Autodesk Inventor part; units mm, degrees
ref_plane "Lock Pin Hole Plane" through (0, 0, 12.7) normal (0, 0, 1) x (1, 0, 0)
ref_plane "YZ Plane" through (0, 0, 0) normal (1, 0, 0) x (0, 1, 0)
ref_plane "XZ Plane" through (0, 0, 0) normal (0, 1, 0) x (-1, 0, 0)
sketch "Sketch1" plane through (0, 0, 0) normal (1, 0, 0) x (0, 1, 0)
  circle A0 centre (0, 0) radius 6.19 construction
  circle A1 centre (0, 0) radius 10
  dimension "d0" = 20
  dimension "d1" = 3.81
extrude "Main Shaft" add sketch "Sketch1" against normal blind 50.8
sketch "Sketch2" plane through (0, 0, 0) normal (1, 0, 0) x (0, 0, -1)
  circle A0 centre (0, 0) radius 30
  dimension "d4" = 60
extrude "CV Flange" add sketch "Sketch2" along normal blind 5
sketch "Sketch3" plane through (5, 0, 0) normal (1, 0, 0) x (0, 0, -1)
  circle A0 centre (0, 20) radius 5
  circle A1 centre (0, 0) radius 20 construction
  line L0 (0, 0) -> (0, 20) construction
  dimension "d7" = 40
  dimension "d8" = 10
extrude "CV Bolt Hole" cut sketch "Sketch3" against normal up to surface (5 mm away)
pattern_circular "CV Bolt Pattern" count 6 over 360 about axis through (-10, 0, 0) along (1, 0, 0) of "CV Bolt Hole"
chamfer "Weld_Chamfer" distance 2 angle 45 1 edges at (0, -10, 0)
ref_plane "Lock Pin Hole Plane" through (0, 0, 12.7) normal (0, 0, 1) x (1, 0, 0)
sketch "Sketch5" plane through (-50.8, 0, 0) normal (-1, 0, 0) x (0, 0, 1)
  line L0 (-20, 0) -> (15, 0) construction
  line L1 (0, 14) -> (0, -14) construction
  arc A0 (-13, 2) -> (-13, -2) centre (-13, 0) ccw
  arc A1 (-7, -2) -> (-7, 2) centre (-7, 0) ccw
  line L2 (-13, -2) -> (-7, -2)
  line L3 (-13, 2) -> (-7, 2)
  point P0 (0, 0)
  dimension "d23" = 2
  dimension "d24" = 7
  dimension "d25" = 6
extrude "Key Slot" cut sketch "Sketch5" against normal blind 22
pattern_circular "Circular Pattern2" count 4 over 360 about axis through (-10, 0, 0) along (1, 0, 0) of "Key Slot"
sketch "Sketch6" plane through (-50.8, 0, 0) normal (-1, 0, 0) x (0, 0, 1)
  circle A0 centre (0, 0) radius 5
  arc A1 (-7, -2) -> (-7, 2) centre (-7, 0) ccw
extrude "Extrusion6" add sketch "Sketch6" along normal blind 20
thread "M10x1.5 thread"
equation "\"d1\" = Shaft_Wall_Thickness"
equation "\"d2\" = Shaft_Length"
equation "\"d4\" = Driveshaft_Flange_Diameter"
equation "\"d5\" = Driveshaft_Flange_Thickness"
equation "\"d7\" = CV_Bolt_Pattern_Diameter"
equation "\"d8\" = CV_Bolt_Hole_Diameter"
equation "\"Shaft_Diameter\" = 25.4"
equation "\"Shaft_Wall_Thickness\" = 3.81"
equation "\"Driveshaft_Flange_Diameter\" = 60"
equation "\"Driveshaft_Flange_Thickness\" = 5"
equation "\"CV_Bolt_Hole_Diameter\" = 10"
equation "\"d18\" = 0.5 * Shaft_Diameter"
equation "\"Shaft_Length\" = 50.8"
properties part number "Hub-CV Adapter"
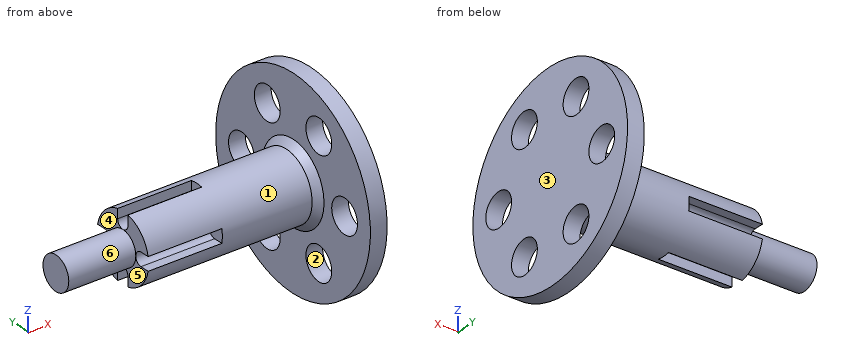
Build history of the part. All positions in model axes, mm. Face numbers are marked on the shaded views. A direction names the side the tool comes from. Round coordinates to 2 decimals unless told otherwise and drop trailing zeros. Loops run counter-clockwise (first coordinate to the right, second up) from the corner with the lowest first, then second, coordinate; pieces in that order, holes last. Notation, with made-up numbers: (-2, 35) -> (24, 35) arc R16 cw to (24, 40) -> close; hole circle Ø11 at (69, 41.25). An arc over 180 degrees is marked (long way). One line per item, written item: value. Start each with the question number.
Q1. Cut at C-C on y = 11. Count the separate pieces of the cut face and the enclosed holes in it, plus the area to 3 significant figures.
Q2. Cut at D-D on z = -25. List the corners of the cut face in (x, y).
Q3. Two-plate mould, pull along Z, no slides. Class the marked faces 1, 2 and 3: released by +Z, released by -Z, zero draft, split by the parting line, or undercut.
Q4. Cut at B-B on y = 20. List the corners of the cut face in (x, z).
Q5. Probe line 1 along Y through (x, z) = (2.75, 0); line 2 along X through (y, z) = (-4.5, 17.5); line 3 along Z through (x, y) = (2, 23). List the from-to ranges inside material, lowest first.
Q6. Drop flat-ended pins along their axis: pin 1 Ø10 at (y, z) = (6, -12.5) entering from -X; pin 2 Ø9 at (y, z) = (10, 17.32) entering from +X; pin 3 Ø2 at (y, z) = (0, 6.5) entering from -X; pin 4 Ø1.4 at (x, z) = (-44.5, -9) entering from +Y. Give the stop position or say it passes through.
Q7. Cut at A-A on x = -42.5. List the corners of the cut face in (y, z).
Q8. 3-axis set-ups, long thin cutter, end or side, ignore diameter. For the marked faces 4, 5 and 6: which of +Z, -Z, +X, -X, +Y, -Y reach the whole face in a straight line?
Computed:
1. separate pieces: 3
1. enclosed holes: 0
1. area: 187 mm²
2. outline: (0, -16.58) -> (5, -16.58) -> (5, 16.58) -> (0, 16.58) -> close
3. face 1: split by the parting line
3. face 2: undercut
3. face 3: zero draft
4. outline: (0, -22.36) -> (5, -22.36) -> (5, -5) -> (0, -5) -> close; (0, 5) -> (5, 5) -> (5, 22.36) -> (0, 22.36) -> close
5. line 1: -30 to -25, -15 to 15, 25 to 30
5. line 2: 0 to 5
5. line 3: -19.26 to -4, 4 to 19.26
6. pin 1: x = -50.8
6. pin 2: through
6. pin 3: x = -28.8
6. pin 4: y = 5.58
7. outline: (-9.8, -2) arc R10 ccw to (-2, -9.8) -> (-2, -7) arc R2 cw to (2, -7) -> (2, -9.8) arc R10 ccw to (9.8, -2) -> (7, -2) arc R2 cw to (7, 2) -> (9.8, 2) arc R10 ccw to (2, 9.8) -> (2, 7) arc R2 cw to (-2, 7) -> (-2, 9.8) arc R10 ccw to (-9.8, 2) -> (-7, 2) arc R2 cw to (-7, -2) -> close
8. face 4: +Z, -X, +Y
8. face 5: -Z, -X, -Y
8. face 6: -X
